from build123d import *

# Parameters (mm, degrees)
SKETCH1_R           = 2.5
SKETCH1_R_2         = 1.5
BOSS_EXTRUDE1_DEPTH = 1.3


with BuildPart() as part:
    # Sketch1 → Boss-Extrude1 (new body)
    with BuildSketch(Plane.XY):
        Polygon((-34.175323676, 43.186140305), (-34.175323676, -17.813859695), (-15.175323676, -36.813859695), (45.824676324, -36.813859695), (64.824676324, -17.813859695), (64.824676324, 43.186140305), (45.824676324, 62.186140305), (-15.175323676, 62.186140305), align=None)
        with Locations((-6.175323676, 18.686140305)):
            Circle(SKETCH1_R, mode=Mode.SUBTRACT)
        with Locations((15.824676324, 18.686140305)):
            Circle(SKETCH1_R, mode=Mode.SUBTRACT)
        with Locations((37.824676324, 18.686140305)):
            Circle(SKETCH1_R, mode=Mode.SUBTRACT)
        with Locations((15.824676324, -22.813859695)):
            Circle(SKETCH1_R, mode=Mode.SUBTRACT)
        with Locations((37.824676324, -22.813859695)):
            Circle(SKETCH1_R, mode=Mode.SUBTRACT)
        with Locations((-6.175323676, -22.813859695)):
            Circle(SKETCH1_R, mode=Mode.SUBTRACT)
        with Locations((-19.175323676, 12.686140305)):
            Circle(SKETCH1_R_2, mode=Mode.SUBTRACT)
        with Locations((-19.175323676, 35.186140305)):
            Circle(SKETCH1_R_2, mode=Mode.SUBTRACT)
        with Locations((50.324676324, 35.186140305)):
            Circle(SKETCH1_R_2, mode=Mode.SUBTRACT)
        with Locations((50.324676324, 12.686140305)):
            Circle(SKETCH1_R_2, mode=Mode.SUBTRACT)
    extrude(amount=BOSS_EXTRUDE1_DEPTH)


solid = part.part
Geometry: final body of the model. Coordinates: model frame, mm. Give positions to 0.01 mm unless a question says otherwise; leave off trailing zeros. Write each loop counter-clockwise with the first axis right and the second up, starting at its lowest first coordinate (ties: lowest second). Pieces come first, ordered by that corner, then holes. Notation, with made-up numbers: (-20, 87.25) -> (37, 87.25) arc R36 cw to (37, 123.25) -> close; hole circle Ø9 at (53.5, 70.5). An arc over 180 degrees is marked (long way). Answer in a Markdown table with one row per item.
(1) Section query C-C on y = 46.5. Return loops of the section in (x, z).
Answers below:
| item | result |
|---|---|
| outline | (-30.86, 0) -> (61.51, 0) -> (61.51, 1.3) -> (-30.86, 1.3) -> close |
(2) Pin query (flat end, axial travel): pin 1 (2.5 mm diameter, centred on x = 50.32, y = 35.19, fed in from -Z). Return the tip coordinate at first contact, or that it passes through.
Answers below:
| item | result |
|---|---|
| pin 1 | through |
(3) Ray query, line 1 along X through (y, z) = (12.5, 0.4); line 2 along X through (y, z) = (18.5, 0.8); line 3 along X through (y, z) = (-24, 0.2). Return the intervals inside material, ascending. Write a range as [from, to].
Answers below:
| item | result |
|---|---|
| line 1 | [-34.18, -20.66], [-17.69, 48.84], [51.81, 64.82] |
| line 2 | [-34.18, -8.67], [-3.68, 13.33], [18.32, 35.33], [40.32, 64.82] |
| line 3 | [-27.99, -8.38], [-3.97, 13.62], [18.03, 35.62], [40.03, 58.64] |
(4) Section query B-B on y = -29.5. Return loops of the section in (x, z).
Answers below:
| item | result |
|---|---|
| outline | (-22.49, 0) -> (53.14, 0) -> (53.14, 1.3) -> (-22.49, 1.3) -> close |
(5) Section query A-A on z = 0.3. State how many separate pieces and enclosed holes the cut face has, then the cut area to 3 significant figures.
Answers below:
| item | result |
|---|---|
| separate pieces | 1 |
| enclosed holes | 10 |
| area | 8,930 mm^2 |
